from build123d import *

# Parameters (mm, degrees)
SKETCH1_W           = 81
SKETCH1_H           = 50
SKETCH1_R           = 2
SKETCH1_R_2         = 1.5
BOSS_EXTRUDE1_DEPTH = 3
CUT_EXTRUDE1_DEPTH  = 4


with BuildPart() as part:
    # Sketch1 → Boss-Extrude1 (new body)
    with BuildSketch(Plane.XY):
        Rectangle(SKETCH1_W, SKETCH1_H)
        with Locations((-34.25, 0)):
            Circle(SKETCH1_R, mode=Mode.SUBTRACT)
        with Locations((-14.25, 0)):
            Circle(SKETCH1_R, mode=Mode.SUBTRACT)
        with Locations((15.75, 0)):
            Circle(SKETCH1_R, mode=Mode.SUBTRACT)
        with Locations((-36.5, 21)):
            Circle(SKETCH1_R_2, mode=Mode.SUBTRACT)
        with Locations((36.5, 21)):
            Circle(SKETCH1_R_2, mode=Mode.SUBTRACT)
        with Locations((36.5, -21)):
            Circle(SKETCH1_R_2, mode=Mode.SUBTRACT)
        with Locations((-36.5, -21)):
            Circle(SKETCH1_R_2, mode=Mode.SUBTRACT)
    extrude(amount=BOSS_EXTRUDE1_DEPTH)

    # Sketch3 → Cut-Extrude1 (cut, through all)
    with BuildSketch(Plane.XY.offset(3)):
        with BuildLine():
            Line((30.5, 18.5), (19, 18.5))
            Line((19, 18.5), (19, 5.629165125))
            ThreePointArc((19, 5.629165125), (20.346194078, 4.596194078), (21.379165125, 3.25))
            Line((21.379165125, 3.25), (34, 3.25))
            Line((34, 3.25), (34, 15))
            ThreePointArc((34, 15), (31.903805922, 16.403805922), (30.5, 18.5))
        make_face()
        with BuildLine():
            Line((12.5, 5.629165125), (12.5, 18.5))
            Line((12.5, 18.5), (-11, 18.5))
            Line((-11, 18.5), (-11, 5.629165125))
            ThreePointArc((-11, 5.629165125), (-9.653805922, 4.596194078), (-8.620834875, 3.25))
            Line((-8.620834875, 3.25), (10.120834875, 3.25))
            ThreePointArc((10.120834875, 3.25), (11.153805922, 4.596194078), (12.5, 5.629165125))
        make_face()
        with BuildLine():
            Line((-28.620834875, 3.25), (-19.879165125, 3.25))
            ThreePointArc((-19.879165125, 3.25), (-18.846194078, 4.596194078), (-17.5, 5.629165125))
            Line((-17.5, 5.629165125), (-17.5, 18.5))
            Line((-17.5, 18.5), (-30.5, 18.5))
            ThreePointArc((-30.5, 18.5), (-31.903805922, 16.403805922), (-34, 15))
            Line((-34, 15), (-34, 6.495190528))
            ThreePointArc((-34, 6.495190528), (-30.892328034, 5.565612183), (-28.620834875, 3.25))
        make_face()
    cut_extrude1 = extrude(amount=-CUT_EXTRUDE1_DEPTH, mode=Mode.SUBTRACT)

    # Mirror2: Cut-Extrude1 across plane
    add(cut_extrude1.mirror(Plane.ZX), mode=Mode.SUBTRACT)


solid = part.part
For this review, take the finished solid that the model builds, in its own axes (mm). Give positions to 0.01 mm unless a question says otherwise; leave off trailing zeros. Loops run counter-clockwise (first coordinate to the right, second up) from the corner with the lowest first, then second, coordinate; pieces in that order, holes last. Notation, with made-up numbers: M 9,84.25 L 43,84.25 A21 ccw 43,109.25 Z; hole C 17,-29 d9. An arc over 180 degrees is marked long. Put each result on its own line as item: value. Start each with the question number.
(1) The part is to be moulded in two halves that separate along X. For faces 1 (the flat face through (-34, 11, 2)), 2 (the flat face through (-1, 0, 3)), say which applies: +X half, -X half, draft (parallel to the pull), parting line (faces both ways), or undercut.
(2) Wall thickness on L1, parallel to X at y = -9.5, z = 1.25; L2, parallel to Y at x = 7, z = 1.8; L3, parallel to Y at x = -36.5, z = 1.4: over which ranges is each line inside the solid? List them lowest first.
(3) Add section B-B, the plane x = 15.75. Write out the cut boundary in (y, z), then the cut area to 3 significant figures.
(4) Add section A-A, the plane y = 0. Write out the cut boundary in (x, z).
(5) For pin 1 (2.5 mm diameter, centred on x = -34.25, y = 0, fed in from +Z), flat-tipped, find the tip position at first contact; note if it passes through.
(6) Add section D-D, the plane x = 36.5. Write out the cut boundary in (y, z), then the cut area to 3 significant figures.
(7) Add section C-C, the plane y = -21. Write out the cut boundary in (x, z), then the cut area to 3 significant figures.
Result:
1. face 1: undercut
1. face 2: draft
2. L1: x = -40.5 to -34, -17.5 to -11, 12.5 to 19, 34 to 40.5
2. L2: y = -25 to -18.5, -3.25 to 3.25, 18.5 to 25
2. L3: y = -25 to -22.5, -19.5 to 19.5, 22.5 to 25
3. outline: M -25,0 L -2,0 L -2,3 L -25,3 Z; M 2,0 L 25,0 L 25,3 L 2,3 Z
3. area: 138 mm^2
4. outline: M -40.5,0 L -36.25,0 L -36.25,3 L -40.5,3 Z; M -32.25,0 L -16.25,0 L -16.25,3 L -32.25,3 Z; M -12.25,0 L 13.75,0 L 13.75,3 L -12.25,3 Z; M 17.75,0 L 40.5,0 L 40.5,3 L 17.75,3 Z
5. pin 1: passes through
6. outline: M -25,0 L -22.5,0 L -22.5,3 L -25,3 Z; M -19.5,0 L 19.5,0 L 19.5,3 L -19.5,3 Z; M 22.5,0 L 25,0 L 25,3 L 22.5,3 Z
6. area: 132 mm^2
7. outline: M -40.5,0 L -38,0 L -38,3 L -40.5,3 Z; M -35,0 L 35,0 L 35,3 L -35,3 Z; M 38,0 L 40.5,0 L 40.5,3 L 38,3 Z
7. area: 225 mm^2
